Study the drawing (mm; zero at the part's minimum x, y, z) and answer. A direction names the side the tool comes from. Coordinates: 2 decimals unless noted, no trailing zeros. Order: outer loops, then holes, each group sorted by start corner. A loop starts at its lowest first (then second) coordinate and runs counter-clockwise, first axis right, second up. Notation, with made-up numbers: M 57.5,19 L 64.5,19 A30 cw 64.5,46 Z; hole C 10,61 d6. An arc over 180 degrees is marked long. Use a Markdown table: item, result. Add a question column.
1) Find section C-C on y = 6. Write down the section's boundary in (x, z), plus the area to 3 significant figures.
2) Find section A-A on z = 13.5. Write down the section's boundary in (x, y), plus the area to 3 significant figures.
3) Find section B-B on x = 7. Write down the section's boundary in (y, z), plus the area to 3 significant figures.
4) For the marked faces 1 and 2, determine the directions among +Z, -Z, +X, -X, +Y, -Y from which every point of the face is accessible in a straight line to the end or side of a thin tool.
5) This flat-tipped pin is pushed along its axis until it touches: pin 1 Ø21 at (x, z) = (37.5, 29.5) entering from -Y (1 decimal). Where does it stop, or does it pass through?
6) The mould has two halves that part along X. Classify the marked faces 3, 4, 5 and 6: released by +X, released by -X, zero draft, split by the parting line, or undercut.
7) Find the intervals of material crossed by probe 1 along X at (y, z) = (8.25, 29.5); probe 2 along Z at (x, y) = (83, 1.75); probe 3 along X at (y, z) = (9.75, 8), in increasing order. Write a range as [from, to].
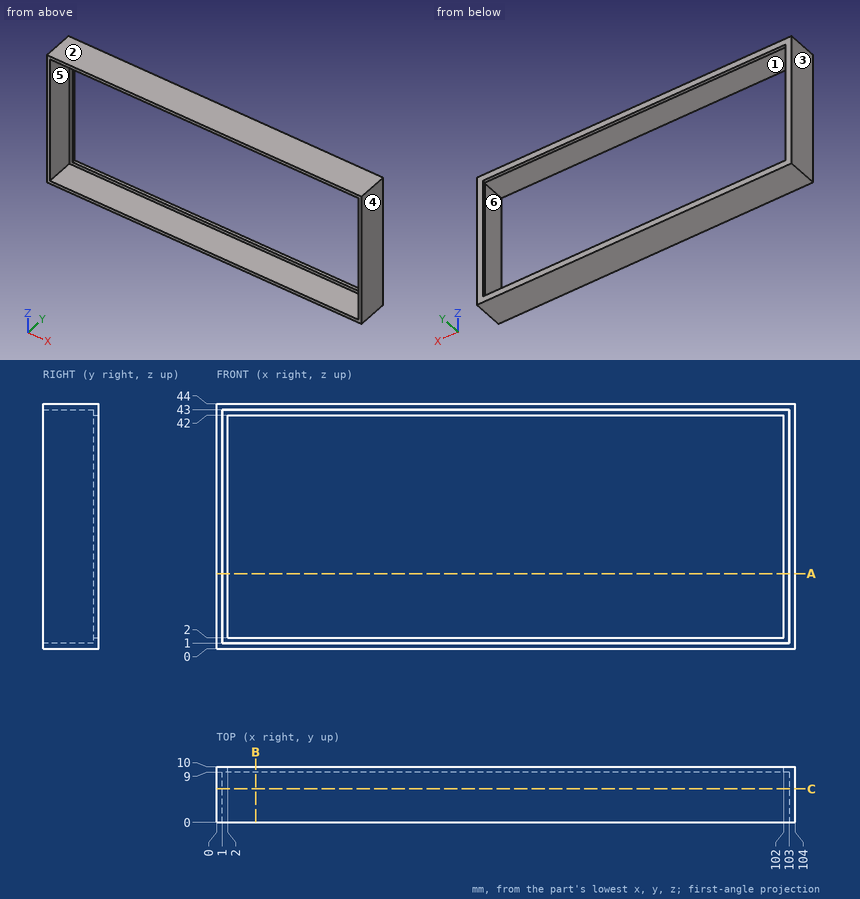
Check result:
| question | item | result |
|---|---|---|
| 1 | outline | M 0,0 L 104,0 L 104,44 L 0,44 Z; hole M 1,1 L 103,1 L 103,43 L 1,43 Z |
| 1 | area | 292 mm2 |
| 2 | outline | M 0,0 L 1,0 L 1,9 L 2,9 L 2,10 L 0,10 Z; M 102,9 L 103,9 L 103,0 L 104,0 L 104,10 L 102,10 Z |
| 2 | area | 22.0 mm2 |
| 3 | outline | M 0,0 L 10,0 L 10,2 L 9,2 L 9,1 L 0,1 Z; M 0,43 L 9,43 L 9,42 L 10,42 L 10,44 L 0,44 Z |
| 3 | area | 22.0 mm2 |
| 4 | face 1 | -Y |
| 4 | face 2 | +Z, +X, -X, +Y, -Y |
| 5 | pin 1 | passes through |
| 6 | face 3 | released by -X |
| 6 | face 4 | released by +X |
| 6 | face 5 | undercut |
| 6 | face 6 | undercut |
| 7 | probe 1 | x = [0, 1], [103, 104] |
| 7 | probe 2 | z = [0, 1], [43, 44] |
| 7 | probe 3 | x = [0, 2], [102, 104] |
